Part model, mm, in its own coordinate system. A direction names the side the tool comes from. Give positions to 0.01 mm unless a question says otherwise; leave off trailing zeros. Write each loop counter-clockwise with the first axis right and the second up, starting at its lowest first coordinate (ties: lowest second). Pieces come first, ordered by that corner, then holes.
from build123d import *

# Parameters (mm, degrees)
SKETCH1_W           = 1549.4
SKETCH1_H           = 76.2
BOSS_EXTRUDE1_DEPTH = 31.75
SKETCH2_R           = 4.7625
CUT_EXTRUDE1_DEPTH  = 777.285876788
SKETCH3_W           = 1422.4
SKETCH3_H           = 95.25
BOSS_EXTRUDE2_DEPTH = 31.75
CHAMFER1_SIZE       = 12.7


with BuildPart() as part:
    # Sketch1 → Boss-Extrude1 (new body)
    with BuildSketch(Plane.XY):
        Rectangle(SKETCH1_W, SKETCH1_H)
    extrude(amount=BOSS_EXTRUDE1_DEPTH)

    # Sketch2 → Cut-Extrude1 (cut, through all)
    with BuildSketch(Plane.XY.offset(31.75)):
        with Locations((742.95, 19.05)):
            Circle(SKETCH2_R)
        with Locations((742.95, -19.05)):
            Circle(SKETCH2_R)
    cut_extrude1 = extrude(amount=-CUT_EXTRUDE1_DEPTH, mode=Mode.SUBTRACT)

    # Mirror1: Cut-Extrude1 across plane
    add(cut_extrude1.mirror(Plane(origin=(0, 0, 0), x_dir=(0, 0, 1), z_dir=(1, 0, 0))), mode=Mode.SUBTRACT)

    # Sketch3 → Boss-Extrude2 (add)
    with BuildSketch(Plane.XY.offset(31.75)):
        with Locations((0, 9.525)):
            Rectangle(SKETCH3_W, SKETCH3_H)
    extrude(amount=BOSS_EXTRUDE2_DEPTH)

    # Chamfer1
    chamfer1_edges = [part.edges().sort_by_distance(p)[0] for p in [
        (0, 57.15, 31.75),
        (0, 57.15, 63.5),
    ]]
    chamfer(chamfer1_edges, length=CHAMFER1_SIZE)


solid = part.part
1) Flat gauge pins, fed straight in: P1, Ø3, axis at y = -14, z = 53, coming from the -X side; P2, Ø5, axis at x = 213, y = 41.5, coming from the -Z side; P3, Ø12.5, axis at x = 742.95, y = -19.05, coming from the +Z side; P4, Ø12.5, axis at x = 742.95, y = 19.05, coming from the -Z side. Where does each tip first touch, or does it go through?
Check result:
P1: stops at x = -711.2
P2: stops at z = 31.75
P3: stops at z = 31.75
P4: stops at z = 0
2) Saw through at A-A (z = 16). State how many separate pieces and enclosed holes the cut face has, and give its area (3 significant figures).
Check result:
separate pieces: 1
enclosed holes: 4
area: 118,000 mm2
3) Drill centre lines: L1, parallel to Y at x = -742.95, z = 23; L2, parallel to X at y = 19, z = 24; L3, parallel to X at y = -16, z = 28.5. Where is each one in solid material? Low to high.
Check result:
L1: y = -38.1 to -23.81, -14.29 to 14.29, 23.81 to 38.1
L2: x = -774.7 to -747.71, -738.19 to 738.19, 747.71 to 774.7
L3: x = -774.7 to -746.61, -739.29 to 739.29, 746.61 to 774.7
4) Saw through at B-B (x = -12). Write the cut outline in (y, z), and give its area (3 significant figures).
Check result:
outline: (-38.1, 0) - (38.1, 0) - (38.1, 31.75) - (44.45, 31.75) - (57.15, 44.45) - (57.15, 50.8) - (44.45, 63.5) - (-38.1, 63.5) - close
area: 5,280 mm2
5) 3-axis set-ups, long thin cutter, end or side, ignore diameter. For faces 1 (the flat face through (-11, -38.1, 31)), 2 (the flat face through (711.2, 9, 47)), 3 (the flat face through (-11, 38.1, 16)), 4 (the flat face through (-743, 1, 31.75)): which of +Z, -Z, +X, -X, +Y, -Y reach the whole face in a straight line?
Check result:
face 1: +Z, -Z, +X, -X, -Y
face 2: +Z, +X, +Y, -Y
face 3: -Z, +X, -X, +Y
face 4: +Z, -X, +Y, -Y
